from build123d import *

# Parameters (mm, degrees)
SKETCH_1_W      = 30
SKETCH_1_H      = 28
EXTRUDE_1_DEPTH = 2
SKETCH_2_W      = 29
SKETCH_2_H      = 19
EXTRUDE_2_DEPTH = 2
SKETCH_3_W      = 29
SKETCH_3_H      = 15
EXTRUDE_3_DEPTH = 2.4


with BuildPart() as part:
    # 草图1 → 凸台-拉伸1 (new body)
    with BuildSketch(Plane.XY):
        Rectangle(SKETCH_1_W, SKETCH_1_H)
    extrude(amount=-EXTRUDE_1_DEPTH)

    # 草图2 → 凸台-拉伸2 (add)
    with BuildSketch(Plane.XY):
        with Locations((0, 0.5)):
            Rectangle(SKETCH_2_W, SKETCH_2_H)
    extrude(amount=EXTRUDE_2_DEPTH)

    # 草图3 → 凸台-拉伸3 (add)
    with BuildSketch(Plane.XY):
        with Locations((0, 2.5)):
            Rectangle(SKETCH_3_W, SKETCH_3_H)
    extrude(amount=EXTRUDE_3_DEPTH)


solid = part.part
Part model, mm, in its own coordinate system. A direction names the side the tool comes from. Coordinates: 2 decimals unless noted, no trailing zeros. Order: outer loops, then holes, each group sorted by start corner. A loop starts at its lowest first (then second) coordinate and runs counter-clockwise, first axis right, second up. Notation, with made-up numbers: M -20,-4.75 L 35,-4.75 A25 ccw 35,16.25 Z; hole C -4.5,-7 d2. An arc over 180 degrees is marked long. Use a Markdown table: item, result.
(1) Flat gauge pins, fed straight in: pin 1 (2.5 mm diameter, centred on x = 1, z = 1.5, fed in from +Y); pin 2 (2 mm diameter, centred on x = -5.5, z = 1.5, fed in from -Y); pin 3 (1.2 mm diameter, centred on x = -5, y = -6.5, fed in from +Z). Where does each tip first touch, or does it go through?
A:
| item | result |
|---|---|
| pin 1 | stops at y = 10 |
| pin 2 | stops at y = -9 |
| pin 3 | stops at z = 2 |
(2) Tool access for faces 4 (the flat face through (0, -14, -1)), 5 (the flat face through (0, -9, 1)), 6 (the flat face through (-14.5, 0, 1)), 7 (the flat face through (0, 10, 1)): list every direction of +Z, -Z, +X, -X, +Y, -Y with a clear straight run to the whole face (end or side of a thin tool).
A:
| item | result |
|---|---|
| face 4 | +Z, -Z, +X, -X, -Y |
| face 5 | +Z, +X, -X, -Y |
| face 6 | +Z, -X, +Y, -Y |
| face 7 | +Z, +X, -X, +Y |
(3) Cut at A-A on y = -5.75. Write the cut outline in (x, z).
A:
| item | result |
|---|---|
| outline | M -15,-2 L 15,-2 L 15,0 L 14.5,0 L 14.5,2 L -14.5,2 L -14.5,0 L -15,0 Z |
(4) Cut at D-D on y = -1.75. Write the cut outline in (x, z).
A:
| item | result |
|---|---|
| outline | M -15,-2 L 15,-2 L 15,0 L 14.5,0 L 14.5,2.4 L -14.5,2.4 L -14.5,0 L -15,0 Z |
(5) Cut at C-C on z = 0.4. Write the cut outline in (x, y), then the cut area to 3 significant figures.
A:
| item | result |
|---|---|
| outline | M -14.5,-9 L 14.5,-9 L 14.5,10 L -14.5,10 Z |
| area | 551 mm^2 |
(6) Probe L1, parallel to Y at x = 13.25, z = 0.7; L2, parallel to X at y = -0.25, z = 0.85; L3, parallel to Z at x = -4, y = -11.5. List the from-to ranges inside material, lowest first.
A:
| item | result |
|---|---|
| L1 | y = -9 to 10 |
| L2 | x = -14.5 to 14.5 |
| L3 | z = -2 to 0 |
(7) Cut at B-B on x = 2.25. Write the cut outline in (y, z).
A:
| item | result |
|---|---|
| outline | M -14,-2 L 14,-2 L 14,0 L 10,0 L 10,2.4 L -5,2.4 L -5,2 L -9,2 L -9,0 L -14,0 Z |
(8) Pull direction Z, two halves, no side cores. Call faces 1 (the flat face through (0, -7, 2)), 2 (the flat face through (0, 0, -2)), 3 (the flat face through (14.5, 0, 1)): released by +Z, released by -Z, zero draft, split by the parting line, or undercut.
A:
| item | result |
|---|---|
| face 1 | released by +Z |
| face 2 | released by -Z |
| face 3 | zero draft |
